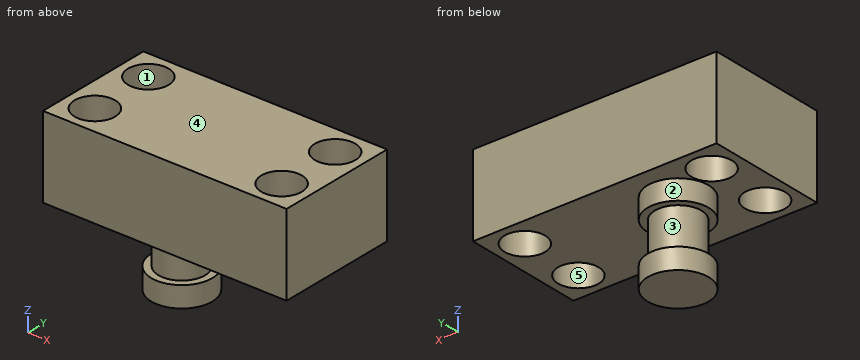
from build123d import *

# Parameters (mm, degrees)
F0_W     = 76.2
F0_H     = 38.1
F1_DEPTH = 25.4
F2_R     = 6.35
F3_DEPTH = 25.4
F4_R     = 9.525
F5_DEPTH = 25.4
F6_W     = 12.7
F6_H     = 12.7


with BuildPart() as f1:
    # F0 (on Top) → F1 (new body)
    with BuildSketch(Plane.XY):
        with Locations((13.890495, -4.273948)):
            Rectangle(F0_W, F0_H)
    extrude(amount=F1_DEPTH)

    # F2 (on Top) → F3 (cut)
    with BuildSketch(Plane.XY):
        with Locations((-15.319505, 5.886052)):
            Circle(F2_R)
        with Locations((-15.319505, -14.433948)):
            Circle(F2_R)
        with Locations((43.100495, 5.886052)):
            Circle(F2_R)
        with Locations((43.100495, -14.433948)):
            Circle(F2_R)
    extrude(amount=F3_DEPTH, mode=Mode.SUBTRACT)

    # F4 (on face) → F5 (join)
    with BuildSketch(Plane(origin=(0, 0, 0), x_dir=(1, 0, 0), z_dir=(0, 0, -1))):
        Circle(F4_R)
    extrude(amount=F5_DEPTH)

    # F6 (on Front) → F7 (revolve, cut)
    with BuildSketch(Plane.XZ):
        with Locations((13.650996, -12.565433)):
            Rectangle(F6_W, F6_H)
    revolve(axis=Axis((0, 0, -25.4), (0, 0, -1)), mode=Mode.SUBTRACT)


solid = f1.part
For this review, take the finished solid that the model builds, in its own axes (mm). Face numbers are marked on the shaded views. A direction names the side the tool comes from. Round coordinates to 2 decimals unless told otherwise and drop trailing zeros. Loops run counter-clockwise (first coordinate to the right, second up) from the corner with the lowest first, then second, coordinate; pieces in that order, holes last. Notation, with made-up numbers: (63.25, 49) - (76.25, 49) arc R29 ccw to (76.25, 72) - close; hole circle Ø2 at (82.5, -0.5). An arc over 180 degrees is marked (long way). Put each result on its own line as item: value. Start each with the question number.
1. Consider section A-A on y = -18. State the section outline as (x, z) points.
2. Consider section D-D on x = 22.5. State the section outline as (y, z) points.
3. Consider section C-C on z = 10.5. State the section outline as (x, y) points.
4. For the marked faces 1 and 2, list the 3-axis set-ups (+Z, -Z, +X, -X, +Y, -Y) from which the entire face can be reached by the end or side of a thin tool; tool diameter is ignored.
5. For probe 1 along X at (y, z) = (6, 8); probe 2 along Z at (x, y) = (-6, 6.5); probe 3 along Y at (x, z) = (48.5, 20), list the stretches that pass through material, from the lowest coordinate up. Write a range as [from, to].
6. Consider section B-B on x = 0. State the section outline as (y, z) points (3 decimals), plus the area to 3 significant figures.
7. Mouldability with a two-part tool opening along X and no side actions: class the marked faces 3, 4 and 5 as +X half, -X half, draft (parallel to the pull), parting line (faces both ways), or undercut.
8. Insertion check: P1, Ø10, axis at y = 8, z = -20, coming from the +X side; P2, Ø14.5, axis at x = 43.1, y = 5.89, coming from the +Z side; P3, Ø10, axis at x = -15.32, y = -14.43, coming from the +Z side; P4, Ø12, axis at x = 7.5, z = -14.5, coming from the -Y side. Each pin has a flat end and moves straight along its axis. Give the tip position at first contact, or say it passes through.
Result sheet:
1. outline: (-24.21, 0) - (-20.57, 0) - (-20.57, 25.4) - (-24.21, 25.4) - close; (-10.07, 0) - (37.85, 0) - (37.85, 25.4) - (-10.07, 25.4) - close; (48.35, 0) - (51.99, 0) - (51.99, 25.4) - (48.35, 25.4) - close
2. outline: (-23.32, 0) - (14.78, 0) - (14.78, 25.4) - (-23.32, 25.4) - close
3. outline: (-24.21, -23.32) - (51.99, -23.32) - (51.99, 14.78) - (-24.21, 14.78) - close; hole circle Ø12.7 at (-15.32, -14.43); hole circle Ø12.7 at (-15.32, 5.89); hole circle Ø12.7 at (43.1, -14.43); hole circle Ø12.7 at (43.1, 5.89)
4. face 1: +Z, -Z
4. face 2: -Z
5. probe 1: [-24.21, -21.67], [-8.97, 36.75], [49.45, 51.99]
5. probe 2: [-25.4, -18.92], [-6.22, 25.4]
5. probe 3: [-23.32, -17.78], [-11.09, 2.54], [9.23, 14.78]
6. outline: (-23.324, 0) - (-9.525, 0) - (-9.525, -6.215) - (-7.301, -6.215) - (-7.301, -18.915) - (-9.525, -18.915) - (-9.525, -25.4) - (9.525, -25.4) - (9.525, -18.915) - (7.301, -18.915) - (7.301, -6.215) - (9.525, -6.215) - (9.525, 0) - (14.776, 0) - (14.776, 25.4) - (-23.324, 25.4) - close
6. area: 1,400 mm^2
7. face 3: parting line
7. face 4: draft
7. face 5: undercut
8. P1: x = 9.04
8. P2: z = 25.4
8. P3: through
8. P4: y = -8.88
